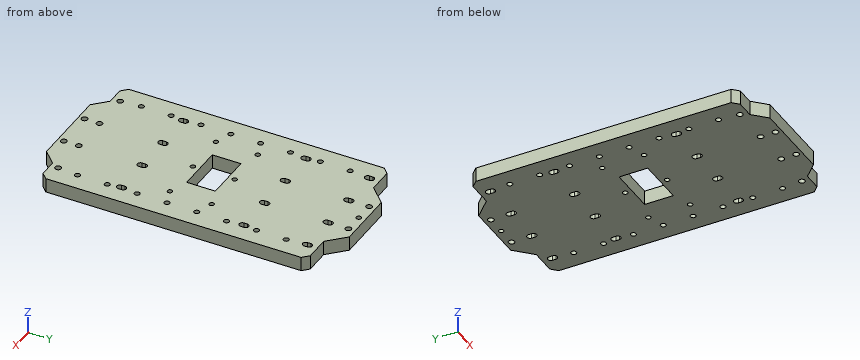
```python
from build123d import *

# Parameters (mm, degrees)
MODEL_R             = 2.5
MODEL_R_2           = 2.05
MODEL_R_3           = 2.25
MODEL_W             = 40
MODEL_H             = 24
BOSS_EXTRUDE1_DEPTH = 12


with BuildPart() as part:
    # Model → Boss-Extrude1 (new body)
    with BuildSketch(Plane.XY):
        Polygon((125, 11), (130, 16), (130, 230), (125, 235), (104, 235), (90, 249), (40, 249), (26, 235), (5, 235), (0, 230), (0, 16), (5, 11), (20, 11), (31, 0), (99, 0), (110, 11), align=None)
        with Locations((16.49, 17.5)):
            Circle(MODEL_R, mode=Mode.SUBTRACT)
        with Locations((48.83, 17.5)):
            Circle(MODEL_R, mode=Mode.SUBTRACT)
        with Locations((81.17, 17.5)):
            Circle(MODEL_R, mode=Mode.SUBTRACT)
        with Locations((113.51, 17.5)):
            Circle(MODEL_R, mode=Mode.SUBTRACT)
        with Locations((29, 139.5)):
            Circle(MODEL_R_2, mode=Mode.SUBTRACT)
        with Locations((65, 139.5)):
            Circle(MODEL_R_2, mode=Mode.SUBTRACT)
        with Locations((101, 139.5)):
            Circle(MODEL_R_2, mode=Mode.SUBTRACT)
        with Locations((101, 104.5)):
            Circle(MODEL_R_2, mode=Mode.SUBTRACT)
        with Locations((65, 104.5)):
            Circle(MODEL_R_2, mode=Mode.SUBTRACT)
        with Locations((29, 104.5)):
            Circle(MODEL_R_2, mode=Mode.SUBTRACT)
        with Locations((65, 243.5)):
            Circle(MODEL_R_2, mode=Mode.SUBTRACT)
        with Locations((81.17, 5)):
            Circle(MODEL_R, mode=Mode.SUBTRACT)
        with Locations((48.83, 5)):
            Circle(MODEL_R, mode=Mode.SUBTRACT)
        with Locations((81.17, 243.5)):
            Circle(MODEL_R, mode=Mode.SUBTRACT)
        with Locations((48.83, 243.5)):
            Circle(MODEL_R, mode=Mode.SUBTRACT)
        with Locations((115, 34.5)):
            Circle(MODEL_R_3, mode=Mode.SUBTRACT)
        with Locations((115, 59.5)):
            Circle(MODEL_R_3, mode=Mode.SUBTRACT)
        with Locations((15, 34.5)):
            Circle(MODEL_R_3, mode=Mode.SUBTRACT)
        with Locations((15, 59.5)):
            Circle(MODEL_R_3, mode=Mode.SUBTRACT)
        with Locations((15, 84.5)):
            Circle(MODEL_R_3, mode=Mode.SUBTRACT)
        with Locations((15, 109.5)):
            Circle(MODEL_R_3, mode=Mode.SUBTRACT)
        with Locations((115, 84.5)):
            Circle(MODEL_R_3, mode=Mode.SUBTRACT)
        with Locations((115, 109.5)):
            Circle(MODEL_R_3, mode=Mode.SUBTRACT)
        with Locations((115, 134.5)):
            Circle(MODEL_R_3, mode=Mode.SUBTRACT)
        with Locations((15, 134.5)):
            Circle(MODEL_R_3, mode=Mode.SUBTRACT)
        with Locations((15, 159.5)):
            Circle(MODEL_R_3, mode=Mode.SUBTRACT)
        with Locations((115, 159.5)):
            Circle(MODEL_R_3, mode=Mode.SUBTRACT)
        with Locations((115, 184.5)):
            Circle(MODEL_R_3, mode=Mode.SUBTRACT)
        with Locations((15, 184.5)):
            Circle(MODEL_R_3, mode=Mode.SUBTRACT)
        with Locations((15, 209.5)):
            Circle(MODEL_R_3, mode=Mode.SUBTRACT)
        with Locations((115, 209.5)):
            Circle(MODEL_R_3, mode=Mode.SUBTRACT)
        with Locations((65, 122)):
            Rectangle(MODEL_W, MODEL_H, mode=Mode.SUBTRACT)
        with BuildLine():
            Line((13.99, 174.82), (13.99, 171.82))
            ThreePointArc((13.99, 171.82), (16.49, 169.32), (18.99, 171.82))
            Line((18.99, 171.82), (18.99, 174.82))
            ThreePointArc((18.99, 174.82), (16.49, 177.32), (13.99, 174.82))
        make_face(mode=Mode.SUBTRACT)
        with BuildLine():
            Line((46.33, 174.82), (46.33, 171.82))
            ThreePointArc((46.33, 171.82), (48.83, 169.32), (51.33, 171.82))
            Line((51.33, 171.82), (51.33, 174.82))
            ThreePointArc((51.33, 174.82), (48.83, 177.32), (46.33, 174.82))
        make_face(mode=Mode.SUBTRACT)
        with BuildLine():
            Line((78.67, 174.82), (78.67, 171.82))
            ThreePointArc((78.67, 171.82), (81.17, 169.32), (83.67, 171.82))
            Line((83.67, 171.82), (83.67, 174.82))
            ThreePointArc((83.67, 174.82), (81.17, 177.32), (78.67, 174.82))
        make_face(mode=Mode.SUBTRACT)
        with BuildLine():
            Line((111.01, 174.82), (111.01, 171.82))
            ThreePointArc((111.01, 171.82), (113.51, 169.32), (116.01, 171.82))
            Line((116.01, 171.82), (116.01, 174.82))
            ThreePointArc((116.01, 174.82), (113.51, 177.32), (111.01, 174.82))
        make_face(mode=Mode.SUBTRACT)
        with BuildLine():
            Line((13.99, 228), (13.99, 225))
            ThreePointArc((13.99, 225), (16.49, 222.5), (18.99, 225))
            Line((18.99, 225), (18.99, 228))
            ThreePointArc((18.99, 228), (16.49, 230.5), (13.99, 228))
        make_face(mode=Mode.SUBTRACT)
        with BuildLine():
            Line((51.33, 225), (51.33, 228))
            ThreePointArc((51.33, 228), (48.83, 230.5), (46.33, 228))
            Line((46.33, 228), (46.33, 225))
            ThreePointArc((46.33, 225), (48.83, 222.5), (51.33, 225))
        make_face(mode=Mode.SUBTRACT)
        with BuildLine():
            Line((83.67, 225), (83.67, 228))
            ThreePointArc((83.67, 228), (81.17, 230.5), (78.67, 228))
            Line((78.67, 228), (78.67, 225))
            ThreePointArc((78.67, 225), (81.17, 222.5), (83.67, 225))
        make_face(mode=Mode.SUBTRACT)
        with BuildLine():
            Line((116.01, 225), (116.01, 228))
            ThreePointArc((116.01, 228), (113.51, 230.5), (111.01, 228))
            Line((111.01, 228), (111.01, 225))
            ThreePointArc((111.01, 225), (113.51, 222.5), (116.01, 225))
        make_face(mode=Mode.SUBTRACT)
        with BuildLine():
            Line((18.99, 69.18), (18.99, 72.18))
            ThreePointArc((18.99, 72.18), (16.49, 74.68), (13.99, 72.18))
            Line((13.99, 72.18), (13.99, 69.18))
            ThreePointArc((13.99, 69.18), (16.49, 66.68), (18.99, 69.18))
        make_face(mode=Mode.SUBTRACT)
        with BuildLine():
            Line((51.33, 69.18), (51.33, 72.18))
            ThreePointArc((51.33, 72.18), (48.83, 74.68), (46.33, 72.18))
            Line((46.33, 72.18), (46.33, 69.18))
            ThreePointArc((46.33, 69.18), (48.83, 66.68), (51.33, 69.18))
        make_face(mode=Mode.SUBTRACT)
        with BuildLine():
            Line((83.67, 69.18), (83.67, 72.18))
            ThreePointArc((83.67, 72.18), (81.17, 74.68), (78.67, 72.18))
            Line((78.67, 72.18), (78.67, 69.18))
            ThreePointArc((78.67, 69.18), (81.17, 66.68), (83.67, 69.18))
        make_face(mode=Mode.SUBTRACT)
        with BuildLine():
            Line((116.01, 69.18), (116.01, 72.18))
            ThreePointArc((116.01, 72.18), (113.51, 74.68), (111.01, 72.18))
            Line((111.01, 72.18), (111.01, 69.18))
            ThreePointArc((111.01, 69.18), (113.51, 66.68), (116.01, 69.18))
        make_face(mode=Mode.SUBTRACT)
    extrude(amount=BOSS_EXTRUDE1_DEPTH)


solid = part.part
```
Can you work these out from the model? Positions are in its coordinate system, mm. Give positions to 0.01 mm unless a question says otherwise; leave off trailing zeros. Order: outer loops, then holes, each group sorted by start corner. A loop starts at its lowest first (then second) coordinate and runs counter-clockwise, first axis right, second up. Notation, with made-up numbers: M 48,65.25 L 66,65.25 A23 ccw 66,93.25 Z; hole C 79,-24 d10. An arc over 180 degrees is marked long. Write item = value, one per line. Start each with the question number.
Q1. Will these pins go through, and if not, where does the flat tip stop? pin 1 Ø3.5 at (x, z) = (114.5, 7.5) entering from -Y; pin 2 Ø4 at (x, z) = (96, 9.5) entering from +Y.
Q2. I need wall thicknesses on probe 1 along X at (y, z) = (85, 5.25); probe 2 along Y at (x, z) = (65, 3.5); probe 3 along Y at (x, z) = (29, 6.5). Which ranges of each line are inside material? Lowest first, please. Write a range as [from, to].
Q3. Suppose I cut it at A-A (y = 84.5). Write out the boundary of the cut face in (x, z).
Q4. Suppose I cut it at B-B (z = 7.25). Count the separate pieces of the cut face and the enclosed holes in it, plus the area to 3 significant figures.
Check result:
q1.pin_1 = 11
q1.pin_2 = 245
q2.probe_1 = [0, 12.81], [17.19, 112.81], [117.19, 130]
q2.probe_2 = [0, 102.45], [106.55, 110], [134, 137.45], [141.55, 241.45], [245.55, 249]
q2.probe_3 = [2, 102.45], [106.55, 137.45], [141.55, 238]
q3.outline = M 0,0 L 12.75,0 L 12.75,12 L 0,12 Z; M 17.25,0 L 112.75,0 L 112.75,12 L 17.25,12 Z; M 117.25,0 L 130,0 L 130,12 L 117.25,12 Z
q4.separate_pieces = 1
q4.enclosed_holes = 44
q4.area = 29,000 mm2
